```python
from build123d import *

# Parameters (mm, degrees)
BOSS_EXTRUDE1_DEPTH = 31.57982
SKETCH2_R           = 13.372801857
CUT_EXTRUDE1_DEPTH  = 117.170888451


with BuildPart() as part:
    # Sketch1 → Boss-Extrude1 (new body)
    with BuildSketch(Plane(origin=(0, 0, 0), x_dir=(1, 0, 0), z_dir=(0, 1, 0))):
        with BuildLine():
            Line((136.250172, 107.259882), (136.250172, 64.988694))
            ThreePointArc((136.250172, 64.988694), (126.511558, 38.118796), (116.772944, 64.988694))
            Line((116.772944, 64.988694), (116.772944, 107.259882))
            Line((116.772944, 107.259882), (119.334788, 108.979208))
            Line((119.334788, 108.979208), (119.334788, 63.925704))
            ThreePointArc((119.334788, 63.925704), (126.511558, 40.670734), (133.688328, 63.925704))
            Line((133.688328, 63.925704), (133.688328, 108.979208))
            Line((133.688328, 108.979208), (136.250172, 107.259882))
        make_face()
    extrude(amount=-BOSS_EXTRUDE1_DEPTH)

    # Sketch2 → Cut-Extrude1 (cut, through all)
    with BuildSketch(Plane(origin=(136.250172, 0, 0), x_dir=(0, 0, -1), z_dir=(1, 0, 0))):
        with Locations((86.524338, -16.195802)):
            Circle(SKETCH2_R)
    extrude(amount=-CUT_EXTRUDE1_DEPTH, mode=Mode.SUBTRACT)


solid = part.part
```
The listing builds one solid part. Answer for the finished solid, in the listing's coordinates (mm). A direction names the side the tool comes from. Coordinates: 2 decimals unless noted, no trailing zeros. Loops run counter-clockwise (first coordinate to the right, second up) from the corner with the lowest first, then second, coordinate; pieces in that order, holes last. Notation, with made-up numbers: (48, 73.25) -> (75, 73.25) arc R21 cw to (75, 83.25) -> close; hole circle Ø4 at (-7, -18.5). An arc over 180 degrees is marked (long way). Use one line per item in the form item = value. Start each with the question number.
Item 1: The part is cut by section B-B on y = -14.5. Determine the outline of the cut face in (x, z), then the cut area to 3 significant figures.
Item 2: The part is cut by section D-D on z = -44. Determine the outline of the cut face in (x, y).
Item 3: The mould has two halves that part along Z. Classify faces 6 (the face through (126.06, -15.57, -40.68)), 7 (the face through (135, -15.6, -108.1)), 8 (the face through (127.032, -15.569, -38.128)), 9 (the face through (134, -31.58, -68)): released by +Z, released by -Z, zero draft, split by the parting line, or undercut.
Item 4: A tool of negligible diameter and unlimited length cuts with its end or side. For faces 1 (the face through (119.335, -30, -87)), 2 (the face through (134.99, -24.33, -75.91)), 3 (the face through (116.773, -5, -76)), 4 (the face through (136.25, -30, -86)), 5 (the face through (134, 0, -68)), from which of +Z, -Z, +X, -X, +Y, -Y can it reach the whole face along a straight path? Write none if from no direction.
Item 5: The part is cut by section C-C on x = 126.5. Determine the outline of the cut face in (y, z).
Item 6: Flat-ended cylindrical pins translate along their axes: pin 1 Ø6 at (y, z) = (-16, -69.5) entering from +X; pin 2 Ø6 at (x, y) = (133, -8.5) entering from +Z; pin 3 Ø5 at (x, y) = (115, -15) entering from -Z. Find the tip coordinate at first contact, or state that the pin passes through.
Item 7: The part is cut by section A-A on z = -102. Determine the outline of the cut face in (x, y), then the cut area to 3 significant figures.
Item 8: Consider L1, parallel to X at y = -4, z = -66; L2, parallel to X at y = -12.5, z = -53; L3, parallel to Z at x = 117, y = -19.5. Determine where each line is inside the solid, lowest interval first. Write a range as [from, to].
Answer key:
q1.outline = (116.77, -107.26) -> (119.33, -108.98) -> (119.33, -99.79) -> (116.77, -99.79) -> close; (116.77, -73.26) -> (119.33, -73.26) -> (119.33, -63.93) arc R12.73 cw (long way) to (133.69, -63.93) -> (133.69, -73.26) -> (136.25, -73.26) -> (136.25, -64.99) arc R15.2 ccw (long way) to (116.77, -64.99) -> close; (133.69, -108.98) -> (136.25, -107.26) -> (136.25, -99.79) -> (133.69, -99.79) -> close
q1.area = 261 mm2
q2.outline = (114.5, -31.58) -> (117.93, -31.58) -> (117.93, 0) -> (114.5, 0) -> close; (135.1, -31.58) -> (138.52, -31.58) -> (138.52, 0) -> (135.1, 0) -> close
q3.face_6 = undercut
q3.face_7 = released by -Z
q3.face_8 = split by the parting line
q3.face_9 = zero draft
q4.face_1 = -Z, +Y, -Y
q4.face_2 = +X, -X
q4.face_3 = -Z, -X, +Y, -Y
q4.face_4 = -Z, +X, +Y, -Y
q4.face_5 = +Z, -Z, +X, -X, +Y
q5.outline = (-31.58, -40.67) -> (0, -40.67) -> (0, -38.12) -> (-31.58, -38.12) -> close
q6.pin_1 = 136.25
q6.pin_2 = -38.52
q6.pin_3 = -107.75
q7.outline = (116.77, -31.58) -> (119.33, -31.58) -> (119.33, 0) -> (116.77, 0) -> close; (133.69, -31.58) -> (136.25, -31.58) -> (136.25, 0) -> (133.69, 0) -> close
q7.area = 162 mm2
q8.L1 = [116.77, 119.33], [133.69, 136.25]
q8.L2 = [111.32, 113.78], [139.24, 141.71]
q8.L3 = [-107.41, -99.48], [-73.57, -61.87], [-44.94, -41.46]
